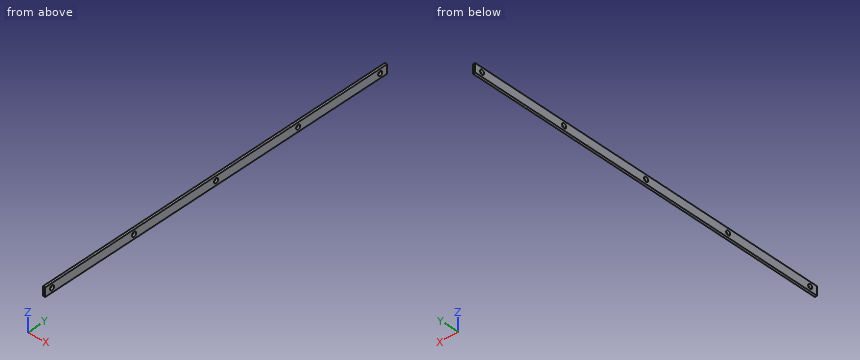
from build123d import *

# Parameters (mm, degrees)
SKETCH1_W           = 12
SKETCH1_H           = 500
BOSS_EXTRUDE1_DEPTH = 3
SKETCH3_R           = 3
CUT_EXTRUDE1_DEPTH  = 3


with BuildPart() as part:
    # Sketch1 → Boss-Extrude1 (new body)
    with BuildSketch(Plane(origin=(0, 0, 0), x_dir=(0, 0, -1), z_dir=(1, 0, 0))):
        Rectangle(SKETCH1_W, SKETCH1_H)
    extrude(amount=BOSS_EXTRUDE1_DEPTH)

    # Sketch3 → Cut-Extrude1 (cut)
    with BuildSketch(Plane.ZY):
        with Locations((0, 240)):
            Circle(SKETCH3_R)
        with Locations((0, 120)):
            Circle(SKETCH3_R)
        Circle(SKETCH3_R)
        with Locations((0, -120)):
            Circle(SKETCH3_R)
        with Locations((0, -240)):
            Circle(SKETCH3_R)
    extrude(amount=-CUT_EXTRUDE1_DEPTH, mode=Mode.SUBTRACT)


solid = part.part
Check sheet for the modelled part. Datum: model origin and axes. Units: mm. Coordinates: 2 decimals unless noted, no trailing zeros. Write each loop counter-clockwise with the first axis right and the second up, starting at its lowest first coordinate (ties: lowest second). Pieces come first, ordered by that corner, then holes. Notation, with made-up numbers: M 30,6.25 L 36,6.25 A22 cw 36,20.25 Z; hole C 85,-38 d6. An arc over 180 degrees is marked long. Answer as CSV lines item,"result".
Q1. Cross-section at B-B (x = 2.45). Record the boundary of the cut face in (y, z).
Check result:
outline,"M -250,-6 L 250,-6 L 250,6 L -250,6 Z; hole C -240,0 d6; hole C -120,0 d6; hole C 0,0 d6; hole C 120,0 d6; hole C 240,0 d6"
Q2. Go/stop test with a flat-tipped pin: pin 1 (3.5 mm diameter, centred on y = -240, z = 0, fed in from +X). Record where the tip stops, or that it passes through.
Check result:
pin 1,"through"
Q3. Material ranges on probe 1 along Y at (x, z) = (1.2, 0.25); probe 2 along Y at (x, z) = (1.35, -1.75); probe 3 along Z at (x, y) = (2, -240), recorded low to high. Write a range as from..to.
Check result:
probe 1,"-250..-242.99, -237.01..-122.99, -117.01..-2.99, 2.99..117.01, 122.99..237.01, 242.99..250"
probe 2,"-250..-242.44, -237.56..-122.44, -117.56..-2.44, 2.44..117.56, 122.44..237.56, 242.44..250"
probe 3,"-6..-3, 3..6"
Q4. Cross-section at A-A (z = 0). Record the boundary of the cut face in (x, y), then the cut area to 3 significant figures.
Check result:
outline,"M 0,-250 L 3,-250 L 3,-243 L 0,-243 Z; M 0,-237 L 3,-237 L 3,-123 L 0,-123 Z; M 0,-117 L 3,-117 L 3,-3 L 0,-3 Z; M 0,3 L 3,3 L 3,117 L 0,117 Z; M 0,123 L 3,123 L 3,237 L 0,237 Z; M 0,243 L 3,243 L 3,250 L 0,250 Z"
area,"1,410 mm^2"
